Source: CAD feature listing. Evaluate the final solid. Frame: model axes, mm. A direction names the side the tool comes from. Give positions to 0.01 mm unless a question says otherwise; leave off trailing zeros. Order: outer loops, then holes, each group sorted by start corner. A loop starts at its lowest first (then second) coordinate and runs counter-clockwise, first axis right, second up. Notation, with made-up numbers: M 77.5,61.5 L 107.5,61.5 A9 cw 107.5,69.5 Z; hole C -20,30 d11. An arc over 180 degrees is marked long. Answer in a Markdown table with one row per item. Add a question column.
(1) Material intervals for line 1 along Z through (x, y) = (0, -15); line 2 along Z through (x, y) = (4, -5); line 3 along Z through (x, y) = (20, -5), sorted ascending.
(2) Section query A-A, the plane y = -34.5. Return loops of the section in (x, z), plus the area to 3 significant figures.
(3) Section query B-B, the plane z = -24.5. Return loops of the section in (x, y).
(4) Set-up query: faces 1 (the face through (5.01, -21.2, 17.07)), 2 (the face through (9, -21, -14)), 3 (the face through (35, -21, -33)). Return all of +Z, -Z, +X, -X, +Y, -Y with unobstructed straight access to the full face (end or side cutting, diameter ignored); none if empty.
(5) Section query C-C, the plane x = 53.5. Return loops of the section in (y, z), plus the area to 3 significant figures.
(6) Mould query, pull axis X, two halves, no side actions, for faces 4 (the face through (-8.58, -21.2, -10.45)), 5 (the face through (26, -21.2, 13.56)), 6 (the face through (65.563, -21.199, 22.522)). Classes: pulls with the +X half, pulls with the -X half, needs draft (parallel to the pull), parting line crosses it, or undercut.
(7) Pin query (flat end, axial travel): P1, Ø3, axis at x = 50.5, y = -7.5, coming from the -Z side; P2, Ø5, axis at x = -2, y = -31.5, coming from the +Z side; P3, Ø8, axis at y = -29, z = 16, coming from the -X side. Return the tip coordinate at first contact, or that it passes through.
from build123d import *

# Parameters (mm, degrees)
F0_R     = 7
F1_DEPTH = 43


with BuildPart() as f1:
    # F0 (on Front) → F1 (new body)
    with BuildSketch(Plane.XZ):
        with BuildLine():
            Line((-14, 11), (-14, -7))
            Line((-14, -7), (-3, -14))
            Line((-3, -14), (21.084766, -14))
            Line((21.084766, -14), (54.69697, -14))
            Line((54.69697, -14), (67, 0))
            Line((67, 0), (67, 21.08522))
            Line((67, 21.08522), (64.08522, 24))
            Line((64.08522, 24), (38, 24))
            ThreePointArc((38, 24), (25.772542, 13.493046), (9.873626, 16.163489))
            Line((9.873626, 16.163489), (0, 18))
            Line((0, 18), (-6.802686, 18.063724))
            Line((-6.802686, 18.063724), (-14, 11))
        make_face()
        Circle(F0_R, mode=Mode.SUBTRACT)
        with BuildLine():
            Line((54.69697, -14), (21.084766, -14))
            ThreePointArc((21.084766, -14), (24.495507, -15.34393), (26.072729, -18.653261))
            ThreePointArc((26.072729, -18.653261), (28.431843, -26.294028), (32.788067, -33))
            Line((32.788067, -33), (38, -33))
            Line((38, -33), (54.69697, -14))
        make_face()
    extrude(amount=F1_DEPTH)


solid = f1.part
Values follow:
| question | item | result |
|---|---|---|
| 1 | line 1 | z = -14 to -7, 7 to 18 |
| 1 | line 2 | z = -14 to -5.74, 5.74 to 17.26 |
| 1 | line 3 | z = -14 to 12.81 |
| 2 | outline | M -14,-7 L -3,-14 L 21.08,-14 A5 cw 26.07,-18.65 A29 ccw 32.79,-33 L 38,-33 L 67,0 L 67,21.09 L 64.09,24 L 38,24 A19 cw 9.87,16.16 L 0,18 L -6.8,18.06 L -14,11 Z; hole C 0,0 d14 |
| 2 | area | 2,720 mm² |
| 3 | outline | M 27.66,-43 L 45.47,-43 L 45.47,0 L 27.66,0 Z |
| 4 | face 1 | +Z, +Y, -Y |
| 4 | face 2 | -Z, -X, +Y, -Y |
| 4 | face 3 | -Z, +X, -X, +Y, -Y |
| 5 | outline | M -43,-15.36 L 0,-15.36 L 0,24 L -43,24 Z |
| 5 | area | 1,690 mm² |
| 6 | face 4 | pulls with the -X half |
| 6 | face 5 | undercut |
| 6 | face 6 | pulls with the +X half |
| 7 | P1 | stops at z = -20.48 |
| 7 | P2 | stops at z = 18.04 |
| 7 | P3 | stops at x = -12.98 |
